Source: CAD feature listing. Evaluate the final solid. Frame: model axes, mm. A direction names the side the tool comes from. Coordinates: 2 decimals unless noted, no trailing zeros. Loops run counter-clockwise (first coordinate to the right, second up) from the corner with the lowest first, then second, coordinate; pieces in that order, holes last. Notation, with made-up numbers: M 84,81 L 102,81 A34 cw 102,111 Z; hole C 50,23 d3. An arc over 180 degrees is marked long. One line per question, with ' | ' between items. Start each with the question number.
1. Section query D-D, the plane y = 16. Output: boundary loops of the cut face in (x, z), and give its area (3 significant figures).
2. Mould query, pull axis Y, two halves, no side actions, for faces 1 (the flat face through (12.3, 50, -0.5)), 2 (the flat face through (-10.07, 47.451, 6.216)), 3 (the flat face through (-10, 0, 2)), 4 (the cylindrical face through (-11, 66, 0)). Classes: pulls with the +Y half, pulls with the -Y half, needs draft (parallel to the pull), parting line crosses it, or undercut.
3. Pin query (flat end, axial travel): P1, Ø3, axis at x = 1, z = -8, coming from the -Y side; P2, Ø2, axis at y = 37, z = -2.5, coming from the -X side; P3, Ø0.6, axis at x = -12, z = 1, coming from the +Y side; P4, Ø1, axis at x = -4.5, y = 9, coming from the +Z side. Return the tip coordinate at first contact, or that it passes through.
4. Section query C-C, the plane z = -8.75. Output: boundary loops of the cut face in (x, y).
5. Section query B-B, the plane y = 66.5. Output: boundary loops of the cut face in (x, z).
6. Ray query, probe 1 along X at (y, z) = (25.5, -0.5); probe 2 along Z at (x, y) = (3.5, 23); probe 3 along X at (y, z) = (36.5, -2.5). Return the intervals inside material, ascending.
7. Section query A-A, the plane x = 0. Output: boundary loops of the cut face in (y, z), and give its area (3 significant figures).
8. Access query for faces 5 (the flat face through (-10.001, 47.451, -6.265)), 6 (the flat face through (-12.2, 45, -0.5)), 7 (the flat face through (12.3, 45, -0.5)), 8 (the flat face through (-11.9, 65, -1)), 9 (the cylindrical face through (-11.427, 67.251, -2.385)). Directions: +Z, -Z, +X, -X, +Y, -Y. A direction counts if a zero-diameter tool reaches every point of the face in a straight line with its end or side. Return the directions, or none.
```python
from build123d import *

# Parameters (mm, degrees)
CROQUIS1_R                 = 11
CROQUIS1_R_2               = 10
SALIENTE_EXTRUIR1_DEPTH    = 70
SALIENTE_EXTRUIR2_START    = -5
SALIENTE_EXTRUIR2_DEPTH    = 5
CORTAR_EXTRUIR1_DEPTH      = 76.139869577
CORTAR_EXTRUIR1_DEPTH_BACK = 76.139869577
REDONDEO1_R                = 1
SALIENTE_EXTRUIR3_START    = -10.5
CROQUIS4_R                 = 2.5
CROQUIS4_R_2               = 1.5
SALIENTE_EXTRUIR3_DEPTH    = 1.4


with BuildPart() as part:
    # Croquis1 → Saliente-Extruir1 (new body)
    with BuildSketch(Plane(origin=(0, 0, 0), x_dir=(1, 0, 0), z_dir=(0, 1, 0))):
        with Locations(Location((0, 0, 0), (0, 0, 270))):
            Circle(CROQUIS1_R)
        with Locations(Location((0, 0, 0), (0, 0, 270))):
            Circle(CROQUIS1_R_2, mode=Mode.SUBTRACT)
    extrude(amount=SALIENTE_EXTRUIR1_DEPTH)

    # Croquis2 → Saliente-Extruir2 (add)
    with BuildSketch(Plane(origin=(0, 50, 0), x_dir=(1, 0, 0), z_dir=(0, 1, 0)).offset(SALIENTE_EXTRUIR2_START)):
        with BuildLine():
            Line((-12.5, 4.5), (-12.5, -4.5))
            Line((-12.5, -4.5), (-7.570478535, -7.980467076))
            ThreePointArc((-7.570478535, -7.980467076), (-11, 0), (-7.570478535, 7.980467076))
            Line((-7.570478535, 7.980467076), (-12.5, 4.5))
        make_face()
        with BuildLine():
            Line((12.5, -4.5), (12.5, 4.5))
            Line((12.5, 4.5), (7.570478535, 7.980467076))
            ThreePointArc((7.570478535, 7.980467076), (11, 0), (7.570478535, -7.980467076))
            Line((7.570478535, -7.980467076), (12.5, -4.5))
        make_face()
    extrude(amount=SALIENTE_EXTRUIR2_DEPTH)

    # Croquis3 → Cortar-Extruir1 (cut, two sides: drawn at the far end of the back side and taken through both)
    with BuildSketch(Plane.ZY.offset(12.5).offset(-CORTAR_EXTRUIR1_DEPTH_BACK)):
        with BuildLine():
            ThreePointArc((0, 49), (-1.5, 47.5), (0, 46))
            Line((0, 46), (0, 49))
        make_face()
        with BuildLine():
            Line((0, 49), (0, 46))
            ThreePointArc((0, 46), (1.060660172, 46.439339828), (1.5, 47.5))
            ThreePointArc((1.5, 47.5), (1.060660172, 48.560660172), (0, 49))
        make_face()
    extrude(amount=CORTAR_EXTRUIR1_DEPTH + CORTAR_EXTRUIR1_DEPTH_BACK, mode=Mode.SUBTRACT)

    # Redondeo1
    redondeo1_edges = [part.edges().sort_by_distance(p)[0] for p in [
        (-11, 50, 0),
        (-11, 45, 0),
        (11, 45, 0),
        (11, 50, 0),
    ]]
    fillet(redondeo1_edges, radius=REDONDEO1_R)

    # Croquis4 → Saliente-Extruir3 (add)
    with BuildSketch(Plane(origin=(0, 0, 0), x_dir=(0, 0, -1), z_dir=(1, 0, 0)).offset(SALIENTE_EXTRUIR3_START)):
        with Locations((0, 66.5)):
            Circle(CROQUIS4_R)
        with Locations((0, 66.5)):
            Circle(CROQUIS4_R_2, mode=Mode.SUBTRACT)
    extrude(amount=-SALIENTE_EXTRUIR3_DEPTH)


solid = part.part
```
Taken from the geometry:
1) outline: C 0,0 d22; hole C 0,0 d20 | area: 66.0 mm^2
2) face 1: pulls with the +Y half | face 2: needs draft | face 3: pulls with the -Y half | face 4: undercut
3) P1: through | P2: x = -10.9 | P3: y = 68.89 | P4: z = 10.25
4) outline: M -6.67,0 L -4.84,0 L -4.84,70 L -6.67,70 Z; M 4.84,0 L 6.67,0 L 6.67,70 L 4.84,70 Z
5) outline: M -11.9,-2.5 L -10.71,-2.5 A11 ccw long -10.71,2.5 L -11.9,2.5 L -11.9,1.5 L -10.9,1.5 A11 ccw -10.9,-1.5 L -11.9,-1.5 Z; hole C 0,0 d20
6) probe 1: -10.99 to -9.99, 9.99 to 10.99 | probe 2: -10.43 to -9.37, 9.37 to 10.43 | probe 3: -10.71 to -9.68, 9.68 to 10.71
7) outline: M 0,-11 L 70,-11 L 70,-10 L 0,-10 Z; M 0,10 L 70,10 L 70,11 L 0,11 Z | area: 140 mm^2
8) face 5: -Z, -X, +Y, -Y | face 6: -X, -Y | face 7: +X, -Y | face 8: +Z, -Z, -X, +Y | face 9: -X
